```python
from build123d import *

# Parameters (mm, degrees)
SKETCH1_W               = 34.036
SKETCH1_H               = 63.5
BOSS_EXTRUDE1_DEPTH     = 21.844
CUT_EXTRUDE1_DEPTH      = 43.12879253
CUT_EXTRUDE1_DEPTH_BACK = 43.12879253
CUT_EXTRUDE2_DEPTH      = 43.12879253
CUT_EXTRUDE2_DEPTH_BACK = 43.12879253
SKETCH3_R               = 2.54
FILLET1_R               = 12.7
FILLET2_R               = 6.35
FILLET3_R               = 1.778
FILLET4_R               = 4.572


with BuildPart() as part:
    # Sketch1 → Boss-Extrude1 (new body)
    with BuildSketch(Plane.XY):
        Rectangle(SKETCH1_W, SKETCH1_H)
    extrude(amount=BOSS_EXTRUDE1_DEPTH)

    # Sketch2 → Cut-Extrude1 (cut, two sides: drawn at the far end of the back side and taken through both)
    with BuildSketch(Plane(origin=(0, 0, 0), x_dir=(1, 0, 0), z_dir=(0, 1, 0)).offset(-CUT_EXTRUDE1_DEPTH_BACK)):
        Polygon((14.224, -108.086321581), (14.224, -21.844), (14.224, -2.794), (-14.224, -2.794), (-14.224, -21.844), (-14.224, -108.086321581), (-14.224, -280.570964742), (14.224, -280.570964742), align=None)
    extrude(amount=CUT_EXTRUDE1_DEPTH + CUT_EXTRUDE1_DEPTH_BACK, mode=Mode.SUBTRACT)

    # Sketch3 → Cut-Extrude2 (cut, two sides: drawn at the far end of the back side and taken through both)
    with BuildSketch(Plane(origin=(0, 0, 0), x_dir=(0, 0, -1), z_dir=(1, 0, 0)).offset(-CUT_EXTRUDE2_DEPTH_BACK)):
        with Locations((-13.2334, 16.1544)):
            Circle(SKETCH3_R)
        with BuildLine():
            Line((-2.2352, 15.3162), (2.957237461, 15.3162))
            Line((2.957237461, 15.3162), (2.957237461, -10.1854))
            Line((2.957237461, -10.1854), (-2.2352, -10.1854))
            ThreePointArc((-2.2352, -10.1854), (-4.031251224, -9.441451224), (-4.7752, -7.6454))
            Line((-4.7752, -7.6454), (-4.7752, 12.7762))
            ThreePointArc((-4.7752, 12.7762), (-4.031251224, 14.572251224), (-2.2352, 15.3162))
        make_face()
        Polygon((-13.208, 31.75), (-21.844, 23.114), (-30.192518149, 23.114), (-30.192518149, 40.531352169), (-13.208, 40.531352169), align=None)
        Polygon((-16.256, -31.889517823), (-16.256, -43.289335124), (-30.986485738, -43.289335124), (-30.986485738, 4.366875898), (-25.970871418, 4.366875898), align=None)
    extrude(amount=CUT_EXTRUDE2_DEPTH + CUT_EXTRUDE2_DEPTH_BACK, mode=Mode.SUBTRACT)

    # Fillet1
    fillet1_edges = [part.edges().sort_by_distance(p)[0] for p in [
        (15.621, 31.75, 13.208),
        (-15.621, 31.75, 13.208),
        (15.621, -11.034817911, 21.844),
        (-15.621, -11.034817911, 21.844),
    ]]
    fillet(fillet1_edges, radius=FILLET1_R)

    # Fillet2
    fillet2_edges = [part.edges().sort_by_distance(p)[0] for p in [
        (15.621, -31.75, 16.293383688),
        (-15.621, -31.75, 16.293383688),
    ]]
    fillet(fillet2_edges, radius=FILLET2_R)

    # Fillet3
    fillet3_edges = [part.edges().sort_by_distance(p)[0] for p in [
        (15.621, 23.114, 21.844),
        (14.224, -20.936584837, 2.794),
        (14.224, 23.501984837, 2.794),
        (-14.224, -20.936584837, 2.794),
        (-14.224, 23.501984837, 2.794),
        (-15.621, 23.114, 21.844),
    ]]
    fillet(fillet3_edges, radius=FILLET3_R)

    # Fillet4
    fillet4_edges = [part.edges().sort_by_distance(p)[0] for p in [
        (17.018, 23.5331, 0),
        (17.018, -20.9677, 0),
        (-17.018, 23.5331, 0),
        (-17.018, -20.9677, 0),
    ]]
    fillet(fillet4_edges, radius=FILLET4_R)


solid = part.part
```
Geometry: final body of the model. Coordinates: model frame, mm. A direction names the side the tool comes from. Coordinates: 2 decimals unless noted, no trailing zeros. Order: outer loops, then holes, each group sorted by start corner. A loop starts at its lowest first (then second) coordinate and runs counter-clockwise, first axis right, second up. Notation, with made-up numbers: (65, 85.25) -> (123, 85.25) arc R12 cw to (123, 97.25) -> close; hole circle Ø4 at (31.25, 11). An arc over 180 degrees is marked (long way). Answer in a Markdown table with one row per item.
Item 1: Contact query for flat-ended pins moving along their axis: P1, Ø6.5, axis at x = 6, y = -20.5, coming from the +Z side; P2, Ø12, axis at x = 4, z = 18, coming from the -Y side; P3, Ø1.4, axis at x = 15.5, y = -0.5, coming from the -Z side. Output: stop coordinate, or through.
Return value:
| item | result |
|---|---|
| P1 | stops at z = 2.79 |
| P2 | passes through |
| P3 | stops at z = 4.78 |
Item 2: Section D-D on y = 17. Output: boundary loops of the cut face in (x, z).
Return value:
| item | result |
|---|---|
| outline | (-17.02, 4.57) arc R4.57 ccw to (-12.45, 0) -> (12.45, 0) arc R4.57 ccw to (17.02, 4.57) -> (17.02, 10.84) -> (14.22, 10.84) -> (14.22, 4.57) arc R1.78 cw to (12.45, 2.79) -> (-12.45, 2.79) arc R1.78 cw to (-14.22, 4.57) -> (-14.22, 10.84) -> (-17.02, 10.84) -> close; (-17.02, 15.63) -> (-14.22, 15.63) -> (-14.22, 21.84) -> (-17.02, 21.84) -> close; (14.22, 15.63) -> (17.02, 15.63) -> (17.02, 21.84) -> (14.22, 21.84) -> close |
Item 3: Section B-B on x = 11.5. Output: boundary loops of the cut face in (y, z), plus the area to 3 significant figures.
Return value:
| item | result |
|---|---|
| outline | (-31.75, 0) -> (-10.19, 0) -> (-10.19, 2.24) arc R2.54 cw to (-10.12, 2.79) -> (-31.75, 2.79) -> close; (15.25, 2.79) arc R2.54 cw to (15.32, 2.24) -> (15.32, 0) -> (31.75, 0) -> (31.75, 2.79) -> close |
| area | 106 mm² |
Item 4: Draft query along Y for faces 4 (the flat face through (0, 23, 2.794)), 5 (the flat face through (-15.64, -19.75, 19.51)), 6 (the cylindrical face through (-0.08, 15.29, 2.61)). Return one class per face: released by +Y, released by -Y, zero draft, split by the parting line, or undercut.
Return value:
| item | result |
|---|---|
| face 4 | zero draft |
| face 5 | released by -Y |
| face 6 | undercut |
Item 5: Section A-A on y = -6. Output: boundary loops of the cut face in (x, z).
Return value:
| item | result |
|---|---|
| outline | (-17.02, 4.78) -> (-14.22, 4.78) -> (-14.22, 21.84) -> (-17.02, 21.84) -> close; (14.22, 4.78) -> (17.02, 4.78) -> (17.02, 21.84) -> (14.22, 21.84) -> close |
Item 6: Access query for faces 1 (the flat face through (0, 24, 0)), 2 (the cylindrical face through (-13.72, -20.03, 3.33)), 3 (the flat face through (16, 2, 4.775)). Directions: +Z, -Z, +X, -X, +Y, -Y. A direction counts if a zero-diameter tool reaches every point of the face in a straight line with its end or side. Return the directions, or none.
Return value:
| item | result |
|---|---|
| face 1 | -Z, +X, -X, +Y, -Y |
| face 2 | +Z, +Y, -Y |
| face 3 | -Z, +X, -X |
Item 7: Section C-C on z = 13.5. Output: boundary loops of the cut face in (x, y), plus the area to 3 significant figures.
Return value:
| item | result |
|---|---|
| outline | (-17.02, -31.4) -> (-14.22, -31.4) -> (-14.22, 13.63) -> (-17.02, 13.63) -> close; (-17.02, 18.68) -> (-14.22, 18.68) -> (-14.22, 30.47) -> (-17.02, 30.47) -> close; (14.22, -31.4) -> (17.02, -31.4) -> (17.02, 13.63) -> (14.22, 13.63) -> close; (14.22, 18.68) -> (17.02, 18.68) -> (17.02, 30.47) -> (14.22, 30.47) -> close |
| area | 318 mm² |
Item 8: Ray query, L1, parallel to X at y = 0.5, z = 9; L2, parallel to Z at x = -11, y = -26; L3, parallel to X at y = -15.5, z = 3.5. Return the intervals inside material, ascending.
Return value:
| item | result |
|---|---|
| L1 | x = -17.02 to -14.22, 14.22 to 17.02 |
| L2 | z = 0 to 2.79 |
| L3 | x = -16.89 to -13.86, 13.86 to 16.89 |
